Design review of the part built by this model. Coordinates are the model's own, in mm. A direction names the side the tool comes from. Give positions to 0.01 mm unless a question says otherwise; leave off trailing zeros. Loops run counter-clockwise (first coordinate to the right, second up) from the corner with the lowest first, then second, coordinate; pieces in that order, holes last. Notation, with made-up numbers: M -14,38 L 14,38 A23 ccw 14,73 Z; hole C 19,11 d9. An arc over 180 degrees is marked long. Use CSV: the item, a comma, the result in double quotes.
Autodesk Inventor part; units mm, degrees
ref_plane "XZ Plane" through (0, 0, 0) normal (0, 1, 0) x (-1, 0, 0)
ref_plane "XY Plane" through (0, 0, 0) normal (0, 0, 1) x (1, 0, 0)
sketch "Sketch1" plane through (0, 0, 0) normal (0, 1, 0) x (-1, 0, 0)
  line L0 (0, 0) -> (0, -270.69) construction
  line L1 (-4, 0) -> (-4, -270.69)
  line L2 (4, -270.69) -> (4, 0)
  arc A0 (4, 0) -> (-4, 0) centre (0, 0) ccw
  arc A1 (-4, -270.69) -> (4, -270.69) centre (0, -270.69) ccw
  circle A2 centre (0, 0) radius 1.5
  circle A3 centre (0, -270.69) radius 1.5
  line L3 (0, -251.19) -> (0, -190.69) construction
  line L4 (1.5, -251.19) -> (1.5, -190.69)
  line L5 (-1.5, -190.69) -> (-1.5, -251.19)
  arc A4 (-1.5, -251.19) -> (1.5, -251.19) centre (0, -251.19) ccw
  arc A5 (1.5, -190.69) -> (-1.5, -190.69) centre (0, -190.69) ccw
  arc A6 (-4, -185.69) -> (-4, -50.69) centre (-700.7379, -118.19) ccw
  arc A7 (4, -185.69) -> (4, -50.69) centre (-692.7379, -118.19) ccw
  point P0 (0, -135.345)
  point P1 (0, -220.94)
  dimension "d0" = 270.69
  dimension "d1" = 8
  dimension "d2" = 3
  dimension "d3" = 3
  dimension "d10" = 3
  dimension "d11" = 19.5
  dimension "d12" = 80
  dimension "d13" = 85
  dimension "d14" = 220
  dimension "d15" = 700
  dimension "d16" = 700
extrude "Extrusion1" add sketch "Sketch1" along normal blind 8 contours A0 L2 A1 L1 A6 | A7 L2
sketch "Sketch2" plane through (0, 0, 0) normal (0, -1, 0) x (1, 0, 0)
  line L0 (4, 0) -> (4, -50.69)
  arc A0 (4, 0) -> (-4, 0) centre (0, 0) ccw
  line L1 (-4, -50.69) -> (-4, 0)
  arc A1 (-4, -50.69) -> (-4, -185.69) centre (692.7379, -118.19) ccw
  line L2 (-4, -270.69) -> (-4, -185.69)
  arc A2 (-4, -270.69) -> (4, -270.69) centre (0, -270.69) ccw
  line L3 (4, -185.69) -> (4, -270.69)
  arc A3 (4, -50.69) -> (4, -185.69) centre (700.7379, -118.19) ccw
  circle A4 centre (0, 0) radius 1.5
  circle A5 centre (0, -270.69) radius 1.5
  arc A6 (-1.5, -251.19) -> (1.5, -251.19) centre (0, -251.19) ccw
  line L4 (-1.5, -190.69) -> (-1.5, -251.19)
  arc A7 (1.5, -190.69) -> (-1.5, -190.69) centre (0, -190.69) ccw
  line L5 (1.5, -251.19) -> (1.5, -190.69)
sketch "Sketch3" plane through (0, 8, 0) normal (0, 1, 0) x (1, 0, 0)
  line L0 (-41.336, 299.9474) -> (32.3712, 299.9474)
  line L1 (32.3712, 299.9474) -> (32.3712, 128.1205)
  line L2 (32.3712, 128.1205) -> (-41.336, 128.1205)
  line L3 (-41.336, 128.1205) -> (-41.336, 299.9474)
  line L4 (-75.6075, 328.1158) -> (61.009, 328.1158)
  line L5 (61.009, 328.1158) -> (61.009, -56.3822)
  line L6 (61.009, -56.3822) -> (-75.6075, -56.3822)
  line L7 (-75.6075, -56.3822) -> (-75.6075, 328.1158)
  point P0 (0, 0)
extrude "Extrusion2" cut sketch "Sketch3" along normal mid plane 20
properties part number "Part_11_p1"
(1) The part is to be moulded in two halves that separate along Z. For faces 3 (the flat face through (-3, 4, -128.12)), 4 (the cylindrical face through (0.03, 3.94, -189.19)), 5 (the flat face through (-4, 4, -229)), say which applies: released by +Z, released by -Z, zero draft, split by the parting line, or undercut.
A:
face 3,"released by +Z"
face 4,"undercut"
face 5,"zero draft"
(2) We need section B-B on z = -248. State the section outline as (x, y) points.
A:
outline,"M -4,0 L -1.5,0 L -1.5,8 L -4,8 Z; M 1.5,0 L 4,0 L 4,8 L 1.5,8 Z"
(3) Wall thickness on line 1 along Z through (x, y) = (0, 2.25); line 2 along X through (y, z) = (3, -206.5); line 3 along X through (y, z) = (4.5, -252): over which ranges is each line inside the solid? List them lowest first. Write a range as [from, to].
A:
line 1,"[-274.69, -272.19], [-269.19, -252.69], [-189.19, -128.12]"
line 2,"[-4, -1.5], [1.5, 4]"
line 3,"[-4, -1.26], [1.26, 4]"
(4) Machinability: for faces 1 (the flat face through (-2, 8, -200)), 2 (the flat face through (-1.5, 4, -221)), which of the approach directions +Z, -Z, +X, -X, +Y, -Y give a long, thin tool a straight path to every point of the face, cutting with its end or side? Answer none if there is none.
A:
face 1,"+Z, -Z, +X, -X, +Y"
face 2,"+Y, -Y"
(5) We need section A-A on y = 6.5. State the section outline as (x, z) points.
A:
outline,"M -7.19,-128.12 A700 ccw -4,-185.69 L -4,-270.69 A4 ccw 4,-270.69 L 4,-185.69 A700 cw 0.81,-128.12 Z; hole C 0,-270.69 d3; hole M -1.5,-251.19 A1.5 ccw 1.5,-251.19 L 1.5,-190.69 A1.5 ccw -1.5,-190.69 Z"
(6) We need section C-C on x = -5.75. State the section outline as (y, z) points.
A:
outline,"M 0,-164.17 L 8,-164.17 L 8,-128.12 L 0,-128.12 Z"
(7) Clearance check with flat-ended pins moving along their axes: P1, Ø2.5, axis at x = 0, z = -270.69, coming from the -Y side; P2, Ø1, axis at y = 6, z = -157.5, coming from the -X side; P3, Ø4, axis at y = 4.5, z = -222.5, coming from the -X side. State where each tip first meets the part, or that it passes through.
A:
P1,"through"
P2,"x = -6.19"
P3,"x = -4"
(8) We need section D-D on z = -174. State the section outline as (x, y) points, then the cut area to 3 significant figures.
A:
outline,"M -5.03,0 L 2.97,0 L 2.97,8 L -5.03,8 Z"
area,"64.0 mm²"
